Design review of the part built by this model. Coordinates are the model's own, in mm. A direction names the side the tool comes from. Give positions to 0.01 mm unless a question says otherwise; leave off trailing zeros. Loops run counter-clockwise (first coordinate to the right, second up) from the corner with the lowest first, then second, coordinate; pieces in that order, holes last. Notation, with made-up numbers: (60.5, 66.5) -> (92.5, 66.5) arc R18 cw to (92.5, 97.5) -> close; hole circle Ø10 at (43, 59.5). An arc over 180 degrees is marked (long way). Answer in a Markdown table with one row per item. Add a question column.
(1) Consider section C-C on y = 0.85. Write out the cut boundary in (x, z).
(2) For line 1 (Z direction, x = 0, y = 1.4); line 2 (Z direction, x = 0.6, y = 0.6); line 3 (X direction, y = 1.55, z = -21), list the stretches that pass through material, from the lowest coordinate up.
(3) For faces 4 (the cylindrical face through (-0.14, -0.99, -3.39)), 5 (the flat face through (-2.5, 1, -13)), list the 3-axis set-ups (+Z, -Z, +X, -X, +Y, -Y) from which the entire face can be reached by the end or side of a thin tool; tool diameter is ignored.
(4) Consider section B-B on x = 0. Write out the cut boundary in (y, z) (3 decimals).
(5) Consider section D-D on y = -0.5. Write out the cut boundary in (x, z) (3 decimals).
(6) Consider section A-A on z = -21. Write out the cut boundary in (x, y), then the cut area to 3 significant figures.
(7) Draft analysis for pull direction X (two halves, no side actions). For faces 1 (the cylindrical face through (-0.672, 0.986, -18.054)), 2 (the cylindrical face through (-0.14, -0.99, 0.61)), 3 (the flat face through (0, 0, -12)), state which applies: +X half, -X half, draft (parallel to the pull), parting line (faces both ways), or undercut.
(8) For pin 1 (2 mm diameter, centred on x = 0, z = -21, fed in from +Y); pin 2 (3 mm diameter, centred on x = 0, z = -25, fed in from +Y); pin 3 (1 mm diameter, centred on x = -1.5, z = -2.5, fed in from -Y), all flat-tipped, find the tip position at first contact; note any pin that passes through.
Autodesk Inventor part; units mm, degrees
ref_plane "YZ Plane" through (0, 0, 0) normal (1, 0, 0) x (0, 1, 0)
ref_plane "XZ Plane" through (0, 0, 0) normal (0, 1, 0) x (-1, 0, 0)
ref_plane "XY Plane" through (0, 0, 0) normal (0, 0, 1) x (1, 0, 0)
sketch "Sketch1" plane through (0, 0, 0) normal (0, 1, 0) x (-1, 0, 0)
  circle A0 centre (0, 0) radius 2.5
  line L0 (0, 0) -> (0, -25)
  line L1 (0, 0) -> (25, 0) construction
  circle A1 centre (0, -25) radius 2.5
  line L2 (2.5, -25) -> (2.5, 0)
  line L3 (-2.5, 0) -> (-2.5, -25)
  circle A2 centre (0, -25) radius 1.25
  circle A3 centre (0, -21) radius 1.25
  circle A4 centre (0, -17) radius 1.25
  dimension "d0" = 5
  dimension "d1" = 25
  dimension "d2" = 90
  dimension "d3" = 5
  dimension "d4" = 2.5
  dimension "d7" = 4
extrude "Extrusion1" add sketch "Sketch1" along normal blind 2 contours A0 | L2 A1 L0 A3 A4 A0 | A0 L0 A4 A3 A1 L3 | A1
sketch "Sketch2" plane through (0, 0, 0) normal (0, -1, 0) x (1, 0, 0)
  circle A0 centre (0, 0) radius 0.625
  line L0 (2.5, 0) -> (2.5, -25)
  circle A1 centre (0, -2) radius 0.625
  circle A2 centre (0, -4) radius 0.625
  dimension "d14" = 1.25
  dimension "d17" = 2
extrude "Extrusion2" add sketch "Sketch2" along normal blind 2
properties part number "Servo Extension Small"
Values follow:
| question | item | result |
|---|---|---|
| 1 | outline | (-2.5, -25) arc R2.5 ccw to (2.5, -25) -> (2.5, 0) arc R2.5 ccw to (-2.5, 0) -> close; hole circle Ø2.5 at (0, -25); hole circle Ø2.5 at (0, -21); hole circle Ø2.5 at (0, -17) |
| 2 | line 1 | -27.5 to -26.25, -23.75 to -22.25, -19.75 to -18.25, -15.75 to 2.5 |
| 2 | line 2 | -27.43 to -26.1, -23.9 to -22.1, -19.9 to -18.1, -15.9 to 2.43 |
| 2 | line 3 | -2.5 to -1.25, 1.25 to 2.5 |
| 3 | face 4 | -Y |
| 3 | face 5 | +Z, -Z, -X, +Y, -Y |
| 4 | outline | (-2, -4.625) -> (0, -4.625) -> (0, -15.75) -> (2, -15.75) -> (2, 2.5) -> (0, 2.5) -> (0, 0.625) -> (-2, 0.625) -> (-2, -0.625) -> (0, -0.625) -> (0, -1.375) -> (-2, -1.375) -> (-2, -2.625) -> (0, -2.625) -> (0, -3.375) -> (-2, -3.375) -> close; (0, -27.5) -> (2, -27.5) -> (2, -26.25) -> (0, -26.25) -> close; (0, -23.75) -> (2, -23.75) -> (2, -22.25) -> (0, -22.25) -> close; (0, -19.75) -> (2, -19.75) -> (2, -18.25) -> (0, -18.25) -> close |
| 5 | outline | circle Ø1.25 at (0, -4); circle Ø1.25 at (0, -2); circle Ø1.25 at (0, 0) |
| 6 | outline | (-2.5, 0) -> (-1.25, 0) -> (-1.25, 2) -> (-2.5, 2) -> close; (1.25, 0) -> (2.5, 0) -> (2.5, 2) -> (1.25, 2) -> close |
| 6 | area | 5.00 mm2 |
| 7 | face 1 | undercut |
| 7 | face 2 | parting line |
| 7 | face 3 | draft |
| 8 | pin 1 | through |
| 8 | pin 2 | y = 2 |
| 8 | pin 3 | y = 0 |
